Could you check a few things on this model? Use its own coordinates, in mm. A direction names the side the tool comes from. Round coordinates to 2 decimals unless told otherwise and drop trailing zeros. Loops run counter-clockwise (first coordinate to the right, second up) from the corner with the lowest first, then second, coordinate; pieces in that order, holes last. Notation, with made-up numbers: (-1, 31.5) - (7, 31.5) arc R23 ccw to (7, 66.5) - close; hole circle Ø4 at (3, 57). An arc over 180 degrees is marked (long way). Use one line per item in the form item = value.
Autodesk Inventor part; units mm, degrees
ref_plane "YZ Plane" through (0, 0, 0) normal (1, 0, 0) x (0, 1, 0)
ref_plane "XZ Plane" through (0, 0, 0) normal (0, 1, 0) x (-1, 0, 0)
ref_plane "XY Plane" through (0, 0, 0) normal (0, 0, 1) x (1, 0, 0)
sketch "Эскиз1" plane through (0, 0, 0) normal (0, 1, 0) x (-1, 0, 0)
  line L0 (0, 0) -> (0, -15)
  line L1 (0, -15) -> (-23.5, -15)
  line L2 (-23.5, -15) -> (-24.7071, -13.7929)
  line L3 (-25.4142, -13.5) -> (-28.4, -13.5)
  line L4 (-35, -20) -> (-90, -20)
  line L5 (-90, -20) -> (-90, -10)
  line L6 (-90, -10) -> (-120, -10)
  line L7 (-120, -10) -> (-120, 0)
  line L8 (-30, -15.1) -> (-30, -15)
  line L9 (-30, -15) -> (-35, -15)
  line L10 (-35, -15) -> (-35, -20)
  line L11 (0, 0) -> (-120, 0)
  line L12 (24, 0) -> (-144, 0)
  arc A0 (-24.7071, -13.7929) -> (-25.4142, -13.5) centre (-25.4142, -14.5) ccw
  arc A1 (-28.4, -13.5) -> (-30, -15.1) centre (-28.4, -15.1) ccw
  point P0 (-25, -13.5)
  point P1 (-30, -13.5)
  dimension "d3" = 45
  dimension "d6" = 5
  dimension "d8" = 30
  dimension "d9" = 35
  dimension "d11" = 55
  dimension "d14" = 15
  dimension "d15" = 13.5
  dimension "d16" = 15
  dimension "d17" = 20
  dimension "d18" = 10
  dimension "d19" = 120
  dimension "d20" = 1
  dimension "d21" = 1.6
revolve "Вращение1" add sketch "Эскиз1" angle 360 about axis through (-10, 0, 0) along (1, 0, 0)
thread "Резьба1"
chamfer "Фаска1" distance 2 angle 45 2 edges at (0, 0, 15) (120, 0, 10)
chamfer "Фаска2" distance 1 angle 45 2 edges at (35, 0, 20) (90, 0, 20)
sketch "Эскиз2" plane through (0, 0, 0) normal (0, 0, 1) x (1, 0, 0)
  line L0 (105, 10) -> (105, 5)
  line L1 (105, 5) -> (120, 5)
  line L2 (120, 5) -> (120, 10)
  line L3 (120, 10) -> (105, 10)
  line L4 (120, 8) -> (120, -8)
  line L5 (90, 10) -> (118, 10)
  line L6 (90, -10) -> (118, -10)
  point P0 (0, 0)
  dimension "d30" = 15
  dimension "d31" = 15
extrude "Выдавливание1" cut sketch "Эскиз2" along normal through all both and the other way through all
sketch "Эскиз3" plane through (0, 0, 0) normal (0, 0, 1) x (1, 0, 0)
  line L0 (50, 20) -> (50, 15)
  line L1 (50, 15) -> (75, 15)
  line L2 (75, 15) -> (75, 20)
  line L3 (75, 20) -> (50, 20)
  line L4 (35, -19) -> (35, 19)
  line L5 (36, 20) -> (89, 20)
  line L6 (36, -20) -> (89, -20)
  point P0 (0, 0)
  dimension "d34" = 35
  dimension "d35" = 15
  dimension "d36" = 25
extrude "Выдавливание2" cut sketch "Эскиз3" along normal through all both and the other way through all
sketch "Эскиз4" plane through (50, 15, -13.2288) normal (0, 1, 0) x (1, 0, 0)
  line L0 (-74, -13.2288) -> (94, -13.2288)
  line L1 (0, 0) -> (0, -26.4575)
  point P0 (-50, -13.2288)
  point P1 (12.5, -13.2288)
  dimension "d39" = 12.5
hole "Отверстие1" at (62.5, 15, 0) direction (0, -1, 0) diameter 5 depth 20 tip angle 120
properties part number "Вал"
1. If we section it at D-D, the plane x = 57: Write out the boundary of the cut face in (y, z).
Solution:
outline = (15, -13.23) - (15, 13.23) arc R20 ccw (long way) to start
2. If we section it at C-C, the plane x = 110.5: Write out the boundary of the cut face in (y, z).
Solution:
outline = (5, -8.66) - (5, 8.66) arc R10 ccw (long way) to start
3. On a 3-axis mill with a long thin cutter (end or side, diameter ignored), from which of +Z, -Z, +X, -X, +Y, -Y can I reach the whole of each face in a straight line? I mean faces 1 (the face through (32.535, 0.66, 14.985)), 2 (the face through (50, 17, 0)), 3 (the face through (12.901, 0.66, 14.985)), 4 (the face through (112, 5, 0)). Say none if no direction works.
Solution:
face_1 = none
face_2 = +Z, -Z, +Y
face_3 = -X
face_4 = +Z, -Z, +X, +Y
4. If we section it at B-B, the plane x = 82.5: Write out the boundary of the cut face in (y, z), plus the area to 3 significant figures.
Solution:
outline = circle Ø40 at (0, 0)
area = 1,260 mm^2
5. We'd pull the mould along X, two halves only. Please class faces 5 (the face through (62.93, -6.193, -0.057)), 6 (the face through (64.72, 4.86, 1.15)), 7 (the face through (105, 7, 0)), 8 (the face through (0.125, 8.871, 9.674)): +X half, -X half, draft (parallel to the pull), parting line (faces both ways), or undercut.
Solution:
face_5 = undercut
face_6 = undercut
face_7 = +X half
face_8 = -X half
6. For P1, Ø12, axis at x = 70, z = -9.5, coming from the +Y side; P2, Ø5, axis at x = 23, y = -6, coming from the +Z side; P3, Ø1, axis at x = 91.5, y = 14, coming from the +Z side; P4, Ø3, axis at x = 62.5, z = 0, coming from the +Y side, each with a flat end and sliding along its axis, tell me the tip position at first contact or that it passes through.
Solution:
P1 = 19.02
P2 = 14.59
P3 = through
P4 = -5.58
7. Please list where these lines run through material, in increasing order: line 1 along X through (y, z) = (7.5, 0); line 2 along X through (y, z) = (3, 0); line 3 along Z through (x, y) = (89, -0.5).
Solution:
line_1 = 0 to 60, 65 to 105
line_2 = 0 to 60, 65 to 120
line_3 = -19.99 to 19.99
